The listing builds one solid part. Answer for the finished solid, in the listing's coordinates (mm). Face numbers are marked on the shaded views. Give positions to 0.01 mm unless a question says otherwise; leave off trailing zeros. Loops run counter-clockwise (first coordinate to the right, second up) from the corner with the lowest first, then second, coordinate; pieces in that order, holes last. Notation, with made-up numbers: (-4, 34.25) - (31, 34.25) arc R22 ccw to (31, 46.25) - close; hole circle Ø10 at (-4.5, -11). An arc over 180 degrees is marked (long way). Write item = value, one per line. Start each with the question number.
1) The mould has two halves that part along Y. Classify the marked faces 1 and 2: +Y half, -Y half, draft (parallel to the pull), parting line (faces both ways), or undercut.
2) The part is cut by section A-A on y = 140. Write down the section's boundary in (x, z).
3) The part is cut by section C-C on x = 167.73. Write down the section's boundary in (y, z), plus the area to 3 significant figures.
4) The part is cut by section D-D on y = 8. State how many separate pieces and enclosed holes the cut face has, plus the area to 3 significant figures.
5) The part is cut by section B-B on x = 130.5. Write down the section's boundary in (y, z).
6) A flat-ended cylindrical pin translates along its axis: P1, Ø3, axis at x = 168.5, y = 16.5, coming from the -Z side. Find the tip coordinate at first contact, or state that the pin passes through.
7) Consider probe 1 along Y at (x, z) = (167.73, 3.35); probe 2 along Y at (x, z) = (23.5, 3.4); probe 3 along X at (y, z) = (78.5, 2.3) (3 decimals). Determine where each line is inside the solid, lowest interval first.
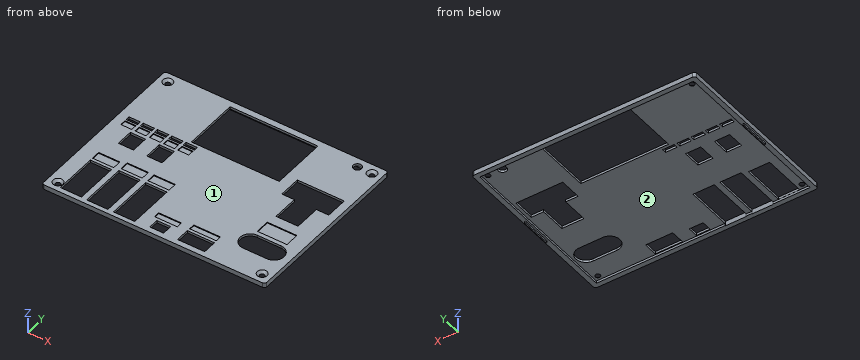
from build123d import *

# Parameters (mm, degrees)
CROQUIS1_W              = 188
CROQUIS1_H              = 148
SALIENTE_EXTRUIR1_DEPTH = 4
CROQUIS2_R              = 2.1
CORTAR_EXTRUIR1_DEPTH   = 4
REDONDEO1_R             = 2
CHAFL_N1_SIZE           = 2
CORTAR_EXTRUIR4_REACH   = 6
CROQUIS4_R              = 3.5
CROQUIS4_W              = 17.9
CROQUIS4_H              = 36.2
CROQUIS4_W_2            = 9.62
CROQUIS4_H_2            = 3.54
CROQUIS4_H_3            = 38.74
CROQUIS4_W_3            = 11.62
CROQUIS4_H_4            = 8.54
CROQUIS4_W_4            = 22.9
CROQUIS4_H_5            = 11.75
CROQUIS4_W_5            = 74
CROQUIS4_H_6            = 46.5
CROQUIS4_W_6            = 12.8
CROQUIS4_H_7            = 14.4
CROQUIS4_H_8            = 14.9
CROQUIS5_W              = 180
CROQUIS5_H              = 140
CORTAR_EXTRUIR5_DEPTH   = 2
SALIENTE_EXTRUIR4_DEPTH = 1.5
CROQUIS8_W              = 17.9
CROQUIS8_H              = 7.5
CROQUIS8_W_2            = 19.22
CROQUIS8_H_2            = 5
CROQUIS8_W_3            = 22.5
CROQUIS8_W_4            = 25
CROQUIS8_H_3            = 12
CROQUIS8_W_5            = 9.22
CROQUIS8_W_6            = 9.222831243
CORTAR_EXTRUIR6_DEPTH   = 0.75


with BuildPart() as part:
    # Croquis1 → Saliente-Extruir1 (new body)
    with BuildSketch(Plane.XY):
        with Locations((94, 74)):
            Rectangle(CROQUIS1_W, CROQUIS1_H)
    extrude(amount=SALIENTE_EXTRUIR1_DEPTH)

    # Croquis2 → Cortar-Extruir1 (cut)
    with BuildSketch(Plane(origin=(0, 0, 0), x_dir=(-1, 0, 0), z_dir=(0, 0, -1))):
        with Locations((-8, 140)):
            Circle(CROQUIS2_R)
        with Locations((-180, 140)):
            Circle(CROQUIS2_R)
        with Locations((-180, 8)):
            Circle(CROQUIS2_R)
        with Locations((-8, 8)):
            Circle(CROQUIS2_R)
    extrude(amount=-CORTAR_EXTRUIR1_DEPTH, mode=Mode.SUBTRACT)

    # Redondeo1
    redondeo1_edges = [part.edges().sort_by_distance(p)[0] for p in [
        (0, 148, 2),
        (188, 148, 2),
        (188, 0, 2),
        (0, 0, 2),
    ]]
    fillet(redondeo1_edges, radius=REDONDEO1_R)

    # Chaflán1
    chafl_n1_edges = [part.edges().sort_by_distance(p)[0] for p in [
        (10.1, 8, 4),
        (182.1, 8, 4),
        (182.1, 140, 4),
        (10.1, 140, 4),
    ]]
    chamfer(chafl_n1_edges, length=CHAFL_N1_SIZE)

    # Croquis4 → Cortar-Extruir4 (cut, up to next)
    with BuildSketch(Plane.XY.offset(4), mode=Mode.PRIVATE) as cortar_extruir4_sk1:
        with Locations((167.73, 140)):
            Circle(CROQUIS4_R)
    cortar_extruir4_tool1 = extrude(cortar_extruir4_sk1.sketch, amount=-CORTAR_EXTRUIR4_REACH, mode=Mode.PRIVATE) & part.part
    add(cortar_extruir4_tool1.solids().sort_by_distance((167.73, 140, 4))[0], mode=Mode.SUBTRACT)
    # Croquis4 → Cortar-Extruir4 (cut, up to next)
    with BuildSketch(Plane.XY.offset(4), mode=Mode.PRIVATE) as cortar_extruir4_sk2:
        with Locations((21.55, 22.21)):
            Rectangle(CROQUIS4_W, CROQUIS4_H)
    cortar_extruir4_tool2 = extrude(cortar_extruir4_sk2.sketch, amount=-CORTAR_EXTRUIR4_REACH, mode=Mode.PRIVATE) & part.part
    add(cortar_extruir4_tool2.solids().sort_by_distance((21.55, 22.21, 4))[0], mode=Mode.SUBTRACT)
    # Croquis4 → Cortar-Extruir4 (cut, up to next)
    with BuildSketch(Plane.XY.offset(4), mode=Mode.PRIVATE) as cortar_extruir4_sk3:
        with Locations((36.44, 92)):
            Rectangle(CROQUIS4_W_2, CROQUIS4_H_2)
    cortar_extruir4_tool3 = extrude(cortar_extruir4_sk3.sketch, amount=-CORTAR_EXTRUIR4_REACH, mode=Mode.PRIVATE) & part.part
    add(cortar_extruir4_tool3.solids().sort_by_distance((36.44, 92, 4))[0], mode=Mode.SUBTRACT)
    # Croquis4 → Cortar-Extruir4 (cut, up to next)
    with BuildSketch(Plane.XY.offset(4), mode=Mode.PRIVATE) as cortar_extruir4_sk4:
        with Locations((44.15, 23)):
            Rectangle(CROQUIS4_W, CROQUIS4_H_3)
    cortar_extruir4_tool4 = extrude(cortar_extruir4_sk4.sketch, amount=-CORTAR_EXTRUIR4_REACH, mode=Mode.PRIVATE) & part.part
    add(cortar_extruir4_tool4.solids().sort_by_distance((44.15, 23, 4))[0], mode=Mode.SUBTRACT)
    # Croquis4 → Cortar-Extruir4 (cut, up to next)
    with BuildSketch(Plane.XY.offset(4), mode=Mode.PRIVATE) as cortar_extruir4_sk5:
        with Locations((66.77, 23)):
            Rectangle(CROQUIS4_W, CROQUIS4_H_3)
    cortar_extruir4_tool5 = extrude(cortar_extruir4_sk5.sketch, amount=-CORTAR_EXTRUIR4_REACH, mode=Mode.PRIVATE) & part.part
    add(cortar_extruir4_tool5.solids().sort_by_distance((66.77, 23, 4))[0], mode=Mode.SUBTRACT)
    # Croquis4 → Cortar-Extruir4 (cut, up to next)
    with BuildSketch(Plane.XY.offset(4), mode=Mode.PRIVATE) as cortar_extruir4_sk6:
        with Locations((93.46, 9)):
            Rectangle(CROQUIS4_W_3, CROQUIS4_H_4)
    cortar_extruir4_tool6 = extrude(cortar_extruir4_sk6.sketch, amount=-CORTAR_EXTRUIR4_REACH, mode=Mode.PRIVATE) & part.part
    add(cortar_extruir4_tool6.solids().sort_by_distance((93.46, 9, 4))[0], mode=Mode.SUBTRACT)
    # Croquis4 → Cortar-Extruir4 (cut, up to next)
    with BuildSketch(Plane.XY.offset(4), mode=Mode.PRIVATE) as cortar_extruir4_sk7:
        with Locations((122.5, 10.525)):
            Rectangle(CROQUIS4_W_4, CROQUIS4_H_5)
    cortar_extruir4_tool7 = extrude(cortar_extruir4_sk7.sketch, amount=-CORTAR_EXTRUIR4_REACH, mode=Mode.PRIVATE) & part.part
    add(cortar_extruir4_tool7.solids().sort_by_distance((122.5, 10.525, 4))[0], mode=Mode.SUBTRACT)
    # Croquis4 → Cortar-Extruir4 (cut, up to next)
    with BuildSketch(Plane.XY.offset(4), mode=Mode.PRIVATE) as cortar_extruir4_sk8:
        with Locations((12.44, 92)):
            Rectangle(CROQUIS4_W_2, CROQUIS4_H_2)
    cortar_extruir4_tool8 = extrude(cortar_extruir4_sk8.sketch, amount=-CORTAR_EXTRUIR4_REACH, mode=Mode.PRIVATE) & part.part
    add(cortar_extruir4_tool8.solids().sort_by_distance((12.44, 92, 4))[0], mode=Mode.SUBTRACT)
    # Croquis4 → Cortar-Extruir4 (cut, up to next)
    with BuildSketch(Plane.XY.offset(4), mode=Mode.PRIVATE) as cortar_extruir4_sk9:
        with Locations((48.44, 92)):
            Rectangle(CROQUIS4_W_2, CROQUIS4_H_2)
    cortar_extruir4_tool9 = extrude(cortar_extruir4_sk9.sketch, amount=-CORTAR_EXTRUIR4_REACH, mode=Mode.PRIVATE) & part.part
    add(cortar_extruir4_tool9.solids().sort_by_distance((48.44, 92, 4))[0], mode=Mode.SUBTRACT)
    # Croquis4 → Cortar-Extruir4 (cut, up to next)
    with BuildSketch(Plane.XY.offset(4), mode=Mode.PRIVATE) as cortar_extruir4_sk10:
        with Locations((24.44, 92)):
            Rectangle(CROQUIS4_W_2, CROQUIS4_H_2)
    cortar_extruir4_tool10 = extrude(cortar_extruir4_sk10.sketch, amount=-CORTAR_EXTRUIR4_REACH, mode=Mode.PRIVATE) & part.part
    add(cortar_extruir4_tool10.solids().sort_by_distance((24.44, 92, 4))[0], mode=Mode.SUBTRACT)
    # Croquis4 → Cortar-Extruir4 (cut, up to next)
    with BuildSketch(Plane.XY.offset(4), mode=Mode.PRIVATE) as cortar_extruir4_sk11:
        with Locations((60.44, 92)):
            Rectangle(CROQUIS4_W_2, CROQUIS4_H_2)
    cortar_extruir4_tool11 = extrude(cortar_extruir4_sk11.sketch, amount=-CORTAR_EXTRUIR4_REACH, mode=Mode.PRIVATE) & part.part
    add(cortar_extruir4_tool11.solids().sort_by_distance((60.44, 92, 4))[0], mode=Mode.SUBTRACT)
    # Croquis4 → Cortar-Extruir4 (cut, up to next)
    with BuildSketch(Plane.XY.offset(4), mode=Mode.PRIVATE) as cortar_extruir4_sk12:
        with Locations((95.52, 119.5)):
            Rectangle(CROQUIS4_W_5, CROQUIS4_H_6)
    cortar_extruir4_tool12 = extrude(cortar_extruir4_sk12.sketch, amount=-CORTAR_EXTRUIR4_REACH, mode=Mode.PRIVATE) & part.part
    add(cortar_extruir4_tool12.solids().sort_by_distance((95.52, 119.5, 4))[0], mode=Mode.SUBTRACT)
    # Croquis4 → Cortar-Extruir4 (cut, up to next)
    with BuildSketch(Plane.XY.offset(4), mode=Mode.PRIVATE) as cortar_extruir4_sk13:
        with Locations((24.425, 73.4)):
            Rectangle(CROQUIS4_W_6, CROQUIS4_H_7)
    cortar_extruir4_tool13 = extrude(cortar_extruir4_sk13.sketch, amount=-CORTAR_EXTRUIR4_REACH, mode=Mode.PRIVATE) & part.part
    add(cortar_extruir4_tool13.solids().sort_by_distance((24.425, 73.4, 4))[0], mode=Mode.SUBTRACT)
    # Croquis4 → Cortar-Extruir4 (cut, up to next)
    with BuildSketch(Plane.XY.offset(4), mode=Mode.PRIVATE) as cortar_extruir4_sk14:
        with Locations((48.425, 73.65)):
            Rectangle(CROQUIS4_W_6, CROQUIS4_H_8)
    cortar_extruir4_tool14 = extrude(cortar_extruir4_sk14.sketch, amount=-CORTAR_EXTRUIR4_REACH, mode=Mode.PRIVATE) & part.part
    add(cortar_extruir4_tool14.solids().sort_by_distance((48.425, 73.65, 4))[0], mode=Mode.SUBTRACT)
    # Croquis4 → Cortar-Extruir4 (cut, up to next)
    with BuildSketch(Plane.XY.offset(4), mode=Mode.PRIVATE) as cortar_extruir4_sk15:
        Polygon((141.84, 104.68), (181.39, 104.68), (181.39, 86.08), (170.94, 86.08), (170.94, 64.08), (152.34, 64.08), (152.34, 86.08), (141.84, 86.08), align=None)
    cortar_extruir4_tool15 = extrude(cortar_extruir4_sk15.sketch, amount=-CORTAR_EXTRUIR4_REACH, mode=Mode.PRIVATE) & part.part
    add(cortar_extruir4_tool15.solids().sort_by_distance((161.623936, 88.12411, 4))[0], mode=Mode.SUBTRACT)
    # Croquis4 → Cortar-Extruir4 (cut, up to next)
    with BuildSketch(Plane.XY.offset(4), mode=Mode.PRIVATE) as cortar_extruir4_sk16:
        with BuildLine():
            Line((153.5, 40), (173.5, 40))
            ThreePointArc((173.5, 40), (182, 31.5), (173.5, 23))
            Line((173.5, 23), (153.5, 23))
            ThreePointArc((153.5, 23), (145, 31.5), (153.5, 40))
        make_face()
    cortar_extruir4_tool16 = extrude(cortar_extruir4_sk16.sketch, amount=-CORTAR_EXTRUIR4_REACH, mode=Mode.PRIVATE) & part.part
    add(cortar_extruir4_tool16.solids().sort_by_distance((163.5, 31.5, 4))[0], mode=Mode.SUBTRACT)

    # Croquis5 → Cortar-Extruir5 (cut)
    with BuildSketch(Plane(origin=(0, 0, 0), x_dir=(-1, 0, 0), z_dir=(0, 0, -1))):
        with Locations((-94, 74)):
            Rectangle(CROQUIS5_W, CROQUIS5_H)
    extrude(amount=-CORTAR_EXTRUIR5_DEPTH, mode=Mode.SUBTRACT)

    # Croquis7 → Saliente-Extruir4 (add)
    with BuildSketch(Plane(origin=(0, 0, 0), x_dir=(-1, 0, 0), z_dir=(0, 0, -1))):
        with BuildLine():
            Line((-186.5, 61.5), (-186.5, 86.5))
            ThreePointArc((-186.5, 86.5), (-186, 87), (-185.5, 86.5))
            Line((-185.5, 86.5), (-185.5, 61.5))
            ThreePointArc((-185.5, 61.5), (-186, 61), (-186.5, 61.5))
        make_face()
        with BuildLine():
            Line((-2.5, 61.5), (-2.5, 86.5))
            ThreePointArc((-2.5, 86.5), (-2, 87), (-1.5, 86.5))
            Line((-1.5, 86.5), (-1.5, 61.5))
            ThreePointArc((-1.5, 61.5), (-2, 61), (-2.5, 61.5))
        make_face()
    extrude(amount=SALIENTE_EXTRUIR4_DEPTH)

    # Croquis8 → Cortar-Extruir6 (cut)
    with BuildSketch(Plane.XY.offset(4)):
        with Locations((21.55, 46.56)):
            Rectangle(CROQUIS8_W, CROQUIS8_H)
        with Locations((44.15, 48.62)):
            Rectangle(CROQUIS8_W, CROQUIS8_H)
        with Locations((66.77, 48.62)):
            Rectangle(CROQUIS8_W, CROQUIS8_H)
        with Locations((93.46, 18.27)):
            Rectangle(CROQUIS8_W_2, CROQUIS8_H_2)
        with Locations((122.5, 21.4)):
            Rectangle(CROQUIS8_W_3, CROQUIS8_H_2)
        with Locations((163.5, 49.5)):
            Rectangle(CROQUIS8_W_4, CROQUIS8_H_3)
        with Locations((12.44, 86.23)):
            Rectangle(CROQUIS8_W_5, CROQUIS8_H_2)
        with Locations((24.44, 86.23)):
            Rectangle(CROQUIS8_W_5, CROQUIS8_H_2)
        with Locations((36.441415621, 86.23)):
            Rectangle(CROQUIS8_W_6, CROQUIS8_H_2)
        with Locations((48.44, 86.23)):
            Rectangle(CROQUIS8_W_5, CROQUIS8_H_2)
        with Locations((60.44, 86.23)):
            Rectangle(CROQUIS8_W_5, CROQUIS8_H_2)
    extrude(amount=-CORTAR_EXTRUIR6_DEPTH, mode=Mode.SUBTRACT)


solid = part.part
Answer below:
q1.face_1 = draft
q1.face_2 = undercut
q2.outline = (0, 0) - (4, 0) - (4, 2) - (5.9, 2) - (3.9, 4) - (0, 4) - close; (10.1, 2) - (58.52, 2) - (58.52, 4) - (12.1, 4) - close; (132.52, 2) - (164.23, 2) - (164.23, 4) - (132.52, 4) - close; (171.23, 2) - (177.9, 2) - (175.9, 4) - (171.23, 4) - close; (182.1, 2) - (184, 2) - (184, 0) - (188, 0) - (188, 4) - (184.1, 4) - close
q3.outline = (0, 0) - (4, 0) - (4, 2) - (23, 2) - (23, 4) - (0, 4) - close; (40, 2) - (64.08, 2) - (64.08, 4) - (55.5, 4) - (55.5, 3.25) - (43.5, 3.25) - (43.5, 4) - (40, 4) - close; (104.68, 2) - (136.5, 2) - (136.5, 4) - (104.68, 4) - close; (143.5, 2) - (144, 2) - (144, 0) - (148, 0) - (148, 4) - (143.5, 4) - close
q3.area = 174 mm2
q4.separate_pieces = 8
q4.enclosed_holes = 0
q4.area = 191 mm2
q5.outline = (0, 0) - (4, 0) - (4, 2) - (4.65, 2) - (4.65, 4) - (0, 4) - close; (16.4, 2) - (96.25, 2) - (96.25, 4) - (23.9, 4) - (23.9, 3.25) - (18.9, 3.25) - (18.9, 4) - (16.4, 4) - close; (142.75, 2) - (144, 2) - (144, 0) - (148, 0) - (148, 4) - (142.75, 4) - close
q6.P1 = 2
q7.probe_1 = 0 to 23, 40 to 43.5, 55.5 to 64.08, 104.68 to 136.5, 143.5 to 148
q7.probe_2 = 0 to 4.11, 40.31 to 42.81, 50.31 to 66.2, 80.6 to 83.73, 88.73 to 90.23, 93.77 to 148
q7.probe_3 = 0 to 18.025, 30.825 to 42.025, 54.825 to 152.34, 170.94 to 188
